For this review, use the dimensioned drawing (mm, ordinates from the lowest corner) and the shaded views. A direction names the side the tool comes from. Round coordinates to 2 decimals unless told otherwise and drop trailing zeros. Write each loop counter-clockwise with the first axis right and the second up, starting at its lowest first coordinate (ties: lowest second). Pieces come first, ordered by that corner, then holes. Notation, with made-up numbers: (-33.75, -31.5) - (-11.75, -31.5) arc R30 ccw to (-11.75, 7.5) - close; hole circle Ø3 at (-24.75, 29). An arc over 180 degrees is marked (long way). Write each question's results on one line, items separated by ' | '.
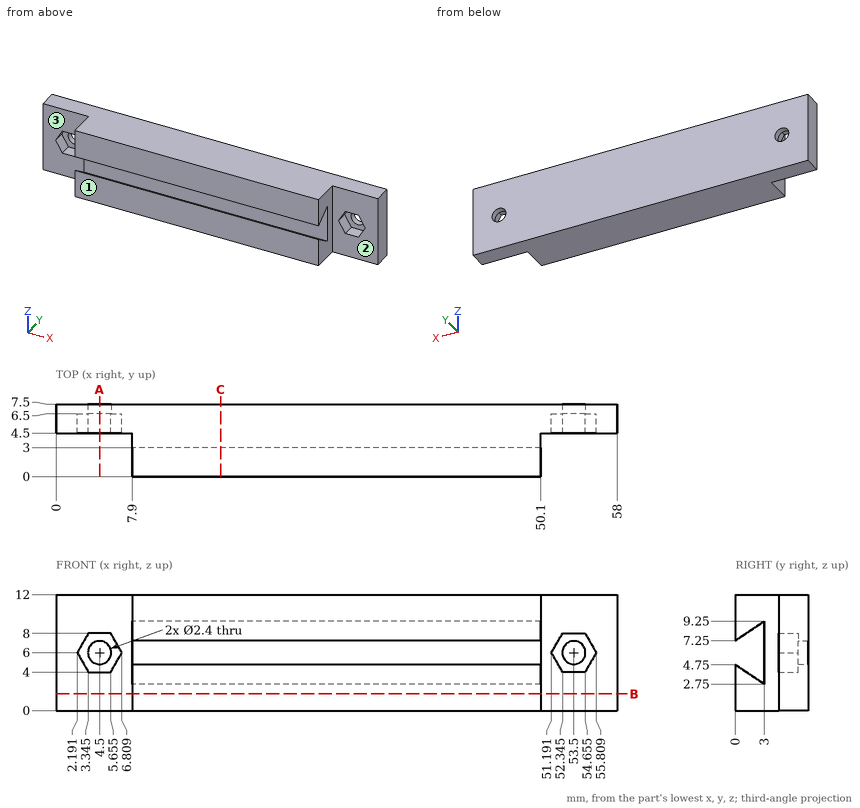
Q1. For probe 1 along X at (y, z) = (7.3, 6); probe 2 along Z at (x, y) = (53.5, 6.75); probe 3 along X at (y, z) = (0.75, 9.75), list the stretches that pass through material, from the lowest coordinate up.
Evaluation:
probe 1: x = 0 to 3.3, 5.7 to 52.3, 54.7 to 58 | probe 2: z = 0 to 4.8, 7.2 to 12 | probe 3: x = 7.9 to 50.1
Q2. We need section C-C (x = 17). State the section outline as (y, z) points, plus the area to 3 significant figures.
Evaluation:
outline: (0, 0) - (7.5, 0) - (7.5, 12) - (0, 12) - (0, 7.25) - (3, 9.25) - (3, 2.75) - (0, 4.75) - close | area: 76.5 mm^2
Q3. Tool access review of the marked faces 1, 2 and 3: name each direction out of +Z, -Z, +X, -X, +Y, -Y from which nothing blocks a thin tool from reaching the whole face with its end or side.
Evaluation:
face 1: +Z, -Z, +X, -X, -Y | face 2: +Z, -Z, +X, -Y | face 3: +Z, -Z, -X, -Y
Q4. Insertion check: P1, Ø3.5, axis at y = 2.5, z = 7.5, coming from the -X side; P2, Ø3, axis at x = 4.5, z = 6, coming from the +Y side; P3, Ø4.5, axis at x = 52.5, z = 5, coming from the -Y side; P4, Ø1.3, axis at y = 2, z = 4.5, coming from the +X side. Each pin has a flat end and moves straight along its axis. Give the tip position at first contact, or say it passes through.
Evaluation:
P1: stops at x = 7.9 | P2: stops at y = 7.5 | P3: stops at y = 4.5 | P4: passes through
Q5. We need section B-B (z = 1.75). State the section outline as (x, y) points.
Evaluation:
outline: (0, 4.5) - (7.9, 4.5) - (7.9, 0) - (50.1, 0) - (50.1, 4.5) - (58, 4.5) - (58, 7.5) - (0, 7.5) - close
Q6. We need section A-A (x = 4.5). State the section outline as (y, z) points.
Evaluation:
outline: (4.5, 0) - (7.5, 0) - (7.5, 4.8) - (6.5, 4.8) - (6.5, 4) - (4.5, 4) - close; (4.5, 8) - (6.5, 8) - (6.5, 7.2) - (7.5, 7.2) - (7.5, 12) - (4.5, 12) - close
